Work out the finished part from the listing and answer in its coordinate system (mm). Face numbers are marked on the shaded views. A direction names the side the tool comes from. Coordinates: 2 decimals unless noted, no trailing zeros. Loops run counter-clockwise (first coordinate to the right, second up) from the corner with the lowest first, then second, coordinate; pieces in that order, holes last. Notation, with made-up numbers: (6.25, -34) - (65.25, -34) arc R15 ccw to (65.25, -21) - close; hole circle Ø6 at (-3, -14). An arc over 180 degrees is marked (long way). Write each question's results on one line, items separated by ' | '. Start each with the question number.
Item 1: Section A-A, the plane z = 0.5 is taken. Write down the section's boundary in (x, y).
Item 2: A tool of negligible diameter and unlimited length cuts with its end or side. For the marked faces 1, 2 and 3, from which of +Z, -Z, +X, -X, +Y, -Y can it reach the whole face along a straight path? Write none if from no direction.
Item 3: Section B-B, the plane x = 8 is taken. Write down the section's boundary in (y, z), plus the area to 3 significant figures.
Item 4: Each of these flat-tipped pins is pushed along its axis until it touches: pin 1 Ø1.8 at (y, z) = (-2, 10) entering from +X; pin 2 Ø1.8 at (x, y) = (8.5, -3) entering from -Z; pin 3 Ø1 at (y, z) = (-3.5, 2) entering from -X; pin 4 Ø1.5 at (y, z) = (-1.5, -14.5) entering from -X. Where does it stop, or does it pass through?
Item 5: For a pull along Z with two mould halves and no side action, classify the marked faces 4, 5, 6 and 7 as +Z half, -Z half, draft (parallel to the pull), parting line (faces both ways), or undercut.
Item 6: Section C-C, the plane y = -4 is taken. Count the separate pieces of the cut face and the enclosed holes in it, plus the area to 3 significant figures.
Item 7: Consider probe 1 along Z at (x, y) = (-15, -1.1); probe 2 along X at (y, z) = (-1.3, 4.5); probe 3 along Z at (x, y) = (-9.5, -2.4). Determine where each line is inside the solid, lowest interval first. Write a range as [from, to].
Item 8: Section D-D, the plane z = 16 is taken. Write down the section's boundary in (x, y), plus the area to 4 significant figures.
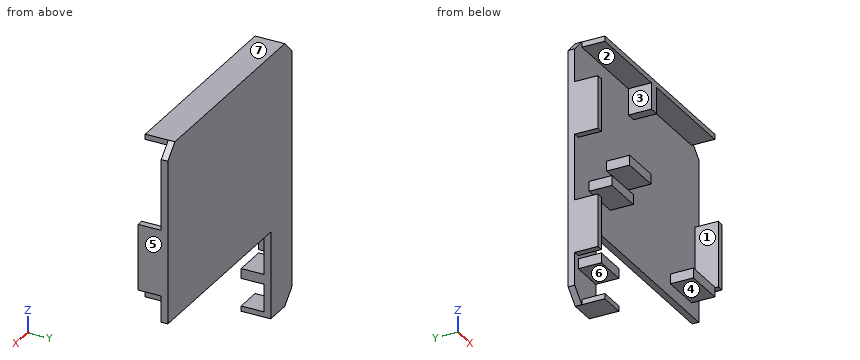
from build123d import *

# Parameters (mm, degrees)
SKETCH_1_W             = 35
SKETCH_1_H             = 40
SM_BASE_FLANGE_1_DEPTH = 1
CHAMFER_1_SIZE         = 2
SKETCH_9_W             = 31
SKETCH_9_H             = 0.8
EXTRUDE_1_DEPTH        = 3.5
CUT_EXTRUDE_1_DEPTH    = 27.804850307
SKETCH_11_W            = 3.944984663
SKETCH_11_H            = 0.8
EXTRUDE_2_DEPTH        = 3.5
SKETCH_12_W            = 1
SKETCH_12_H            = 8
SKETCH_12_H_2          = 10
EXTRUDE_3_DEPTH        = 3.5
SKETCH_13_W            = 6
SKETCH_13_H            = 1.5
SKETCH_13_W_2          = 4.944984663
SKETCH_13_W_3          = 1.5
SKETCH_13_H_2          = 4
EXTRUDE_4_DEPTH        = 3.5


# Sheet-metal steps are written as plain solids
with BuildPart() as part:
    # Sketch 1 → 基体-法兰1 (new body)
    with BuildSketch(Plane(origin=(0, 0, 0), x_dir=(1, 0, 0), z_dir=(0, 1, 0))):
        Rectangle(SKETCH_1_W, SKETCH_1_H)
    extrude(amount=-SM_BASE_FLANGE_1_DEPTH)

    # 倒角1
    chamfer_1_edges = [part.edges().sort_by_distance(p)[0] for p in [
        (17.5, -0.5, 20),
        (-17.5, -0.5, 20),
        (-17.5, -0.5, -20),
        (17.5, -0.5, -20),
    ]]
    chamfer(chamfer_1_edges, length=CHAMFER_1_SIZE)

    # 草图9 → 凸台-拉伸1 (add)
    with BuildSketch(Plane.XZ.offset(1)):
        with Locations((0, 19.6)):
            Rectangle(SKETCH_9_W, SKETCH_9_H)
    extrude(amount=EXTRUDE_1_DEPTH)

    # 草图10 → 切除-拉伸1 (cut, through all)
    with BuildSketch(Plane.XZ.offset(1)):
        Polygon((17.5, -6.777010343), (-11.555015337, -6.777010343), (-11.555015337, -20), (15.5, -20), (17.5, -18), align=None)
    extrude(amount=-CUT_EXTRUDE_1_DEPTH, mode=Mode.SUBTRACT)

    # 草图11 → 凸台-拉伸2 (add)
    with BuildSketch(Plane.XZ.offset(1)):
        with Locations((-13.527507669, -19.6)):
            Rectangle(SKETCH_11_W, SKETCH_11_H)
    extrude(amount=EXTRUDE_2_DEPTH)

    # 草图12 → 凸台-拉伸3 (add)
    with BuildSketch(Plane.XZ.offset(1)):
        with Locations((-17, 9)):
            Rectangle(SKETCH_12_W, SKETCH_12_H)
        with Locations((-17, -9)):
            Rectangle(SKETCH_12_W, SKETCH_12_H)
        with Locations((17, 2.222989657)):
            Rectangle(SKETCH_12_W, SKETCH_12_H_2)
    extrude(amount=EXTRUDE_3_DEPTH)

    # 草图13 → 凸台-拉伸4 (add)
    with BuildSketch(Plane.XZ.offset(1)):
        with Locations((-10.5, -1.027010343)):
            Rectangle(SKETCH_13_W, SKETCH_13_H)
        with Locations((-5.5, 4.472989657)):
            Rectangle(SKETCH_13_W, SKETCH_13_H)
        with Locations((12.5, -4.027010343)):
            Rectangle(SKETCH_13_W, SKETCH_13_H)
        with Locations((-14.027507669, -14.25)):
            Rectangle(SKETCH_13_W_2, SKETCH_13_H)
        with Locations((-1.628117535, 17.2)):
            Rectangle(SKETCH_13_W_3, SKETCH_13_H_2)
    extrude(amount=EXTRUDE_4_DEPTH)


solid = part.part
Answer key:
1) outline: (-17.5, -1) - (16.5, -1) - (16.5, -4.5) - (17.5, -4.5) - (17.5, 0) - (-17.5, 0) - close
2) face 1: +Z, -Z, -Y | face 2: -X, -Y | face 3: -Z, -X, -Y
3) outline: (-4.5, 19.2) - (-1, 19.2) - (-1, -6.78) - (0, -6.78) - (0, 20) - (-4.5, 20) - close | area: 29.6 mm^2
4) pin 1: stops at x = -16.5 | pin 2: stops at z = 19.2 | pin 3: stops at x = 16.5 | pin 4: stops at x = -17.5
5) face 4: -Z half | face 5: draft | face 6: undercut | face 7: +Z half
6) separate pieces: 9 | enclosed holes: 0 | area: 94.4 mm^2
7) probe 1: z = [-20, -19.2], [-15, -13.5], [19.2, 20] | probe 2: x = [-8.5, -2.5], [16.5, 17.5] | probe 3: z = [-1.78, -0.28], [19.2, 20]
8) outline: (-17.5, -1) - (-2.38, -1) - (-2.38, -4.5) - (-0.88, -4.5) - (-0.88, -1) - (17.5, -1) - (17.5, 0) - (-17.5, 0) - close | area: 40.25 mm^2
